The listing builds one solid part. Answer for the finished solid, in the listing's coordinates (mm). Face numbers are marked on the shaded views. Round coordinates to 2 decimals unless told otherwise and drop trailing zeros. Loops run counter-clockwise (first coordinate to the right, second up) from the corner with the lowest first, then second, coordinate; pieces in that order, holes last. Notation, with made-up numbers: M -16.75,38.25 L 40.25,38.25 A35 ccw 40.25,76.25 Z; hole C 52.25,55 d9. An arc over 180 degrees is marked long. Answer as a JSON object with one key per item and string values.
```python
from build123d import *

# Parameters (mm, degrees)
F0_R     = 16
F0_R_2   = 15
F1_DEPTH = 50
F3_DEPTH = 10
F5_W     = 4.5602535829
F5_H     = 2.9019792564
F6_DEPTH = 5
F7_W     = 5.0895041786
F7_H     = 3.3034160733
F8_DEPTH = 49.4


with BuildPart() as f1:
    # F0 (on Top) → F1 (new body)
    with BuildSketch(Plane.XY):
        Circle(F0_R)
        Circle(F0_R_2, mode=Mode.SUBTRACT)
    extrude(amount=F1_DEPTH)

    # F2 (on face) → F3 (cut)
    with BuildSketch(Plane.XY.offset(50)):
        with BuildLine():
            Line((15.9751944562, 0.8905964787), (14.9735379224, 0.8905964787))
            ThreePointArc((14.9735379224, 0.8905964787), (14.9933830211, 0.4454947613), (15, 0))
            ThreePointArc((15, 0), (14.9629845517, -1.0531349891), (14.8521208926, -2.1010723431))
            Line((14.8521208926, -2.1010723431), (15.8614468132, -2.1010723431))
            ThreePointArc((15.8614468132, -2.1010723431), (15.9653241278, -1.0528178827), (16, 0))
            ThreePointArc((16, 0), (15.9937974118, 0.4454709314), (15.9751944562, 0.8905964787))
        make_face()
    extrude(amount=-F3_DEPTH, mode=Mode.SUBTRACT)

    # F5 (on offset) → F6 (cut)
    with BuildSketch(Plane.XY.offset(40)):
        with Locations((14.4062549807, 5.8039587457)):
            Rectangle(F5_W, F5_H)
    extrude(amount=F6_DEPTH, mode=Mode.SUBTRACT)

    # F7 (on Right) → F8 (cut)
    with BuildSketch(Plane.YZ):
        with Locations((2.5447520893, 41.1266498268)):
            Rectangle(F7_W, F7_H)
    extrude(amount=F8_DEPTH, mode=Mode.SUBTRACT)


solid = f1.part
```
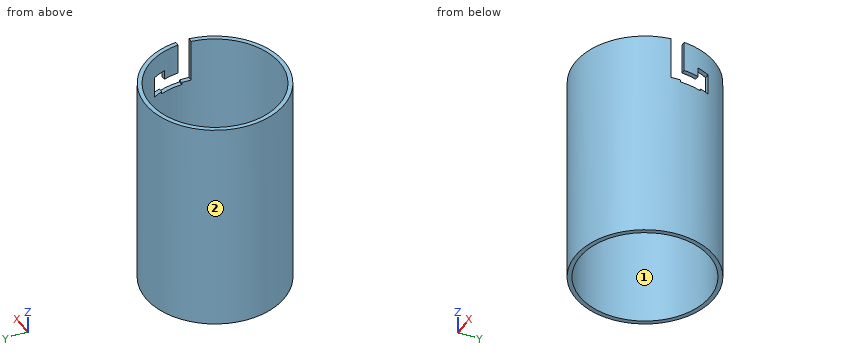
Item 1: The part is cut by section D-D (z = 10.5). Give the vertices of the cut face in (x, y).
Values follow:
{"outline": "C 0,0 d32; hole C 0,0 d30"}
Item 2: Determine the mould class of the marked faces 1 and 2 for opening direction X: released by +X, released by -X, zero draft, split by the parting line, or undercut.
Values follow:
{"face 1": "undercut", "face 2": "split by the parting line"}
Item 3: Straight lines are drawn through the part: line 1 (X direction, y = 0, z = 22); line 2 (Y direction, x = -4, z = 25). For each, find the intervals that lie inside material, in ascending order.
Values follow:
{"line 1": "-16 to -15, 15 to 16", "line 2": "-15.49 to -14.46, 14.46 to 15.49"}
Item 4: The part is cut by section C-C (y = 3). Give the vertices of the cut face in (x, z).
Values follow:
{"outline": "M -15.72,0 L -14.7,0 L -14.7,50 L -15.72,50 Z; M 14.7,0 L 15.72,0 L 15.72,39.47 L 14.7,39.47 Z; M 14.7,42.78 L 15.72,42.78 L 15.72,50 L 14.7,50 Z"}
Item 5: The part is cut by section A-A (x = 0). Give the vertices of the cut face in (y, z), then the cut area to 4 significant figures.
Values follow:
{"outline": "M -16,0 L -15,0 L -15,50 L -16,50 Z; M 15,0 L 16,0 L 16,50 L 15,50 Z", "area": "100.0 mm^2"}
Item 6: The part is cut by section B-B (y = 9). Give the vertices of the cut face in (x, z).
Values follow:
{"outline": "M -13.23,0 L -12,0 L -12,50 L -13.23,50 Z; M 12,0 L 13.23,0 L 13.23,50 L 12,50 Z"}
Item 7: Flat-ended cylindrical pins translate along their axes: P1, Ø0.6, axis at x = 13.5, z = 43, coming from the -Y side; P2, Ø0.6, axis at x = 15.5, y = -0.5, coming from the +Z side; P3, Ø2, axis at y = 1.5, z = 11.5, coming from the +X side. Find the tip coordinate at first contact, or state that the pin passes through.
Values follow:
{"P1": "y = -9.04", "P2": "z = 40", "P3": "x = 15.99"}
